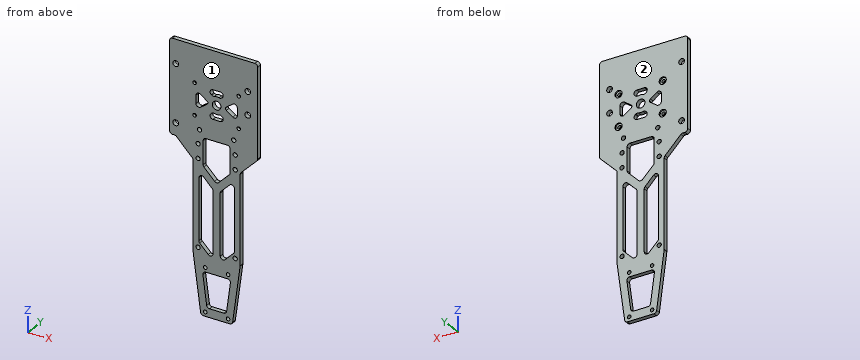
from build123d import *

# Parameters (mm, degrees)
SKETCH_1_R          = 1.25
SKETCH_1_R_2        = 1.5
EXTRUDE_1_DEPTH     = 3
CUT_EXTRUDE_1_DEPTH = 10
FILLET_1_R          = 2
SKETCH_3_R          = 2
CUT_EXTRUDE_2_DEPTH = 185.303255533
SKETCH_5_R          = 1.25
CUT_EXTRUDE_3_DEPTH = 185.303255533
SKETCH_6_R          = 3
CUT_EXTRUDE_4_DEPTH = 10
SKETCH_7_R          = 2.5
CUT_EXTRUDE_5_DEPTH = 1
FILLET_2_R          = 2
SKETCH_8_R          = 1.5
CUT_EXTRUDE_6_DEPTH = 10


with BuildPart() as part:
    # 草图1 → 凸台-拉伸1 (new body)
    with BuildSketch(Plane(origin=(0, 0, 0), x_dir=(1, 0, 0), z_dir=(0, 1, 0))):
        Polygon((11, 0), (-11, 0), (-16.5, -41.3), (-16.5, -104), (-28.8, -116.3), (-33, -116.3), (-33, -181.3), (28.8, -181.3), (28.8, -120.3), (28.8, -116.3), (16.5, -104), (16.5, -41.3), align=None)
        with Locations(Location((-8, -3, 0), (0, 0, 270))):
            Circle(SKETCH_1_R, mode=Mode.SUBTRACT)
        with Locations(Location((-8, -33, 0), (0, 0, 270))):
            Circle(SKETCH_1_R, mode=Mode.SUBTRACT)
        with Locations(Location((8, -33, 0), (0, 0, 90))):
            Circle(SKETCH_1_R, mode=Mode.SUBTRACT)
        with Locations(Location((8, -3, 0), (0, 0, 90))):
            Circle(SKETCH_1_R, mode=Mode.SUBTRACT)
        with Locations(Location((-13, -45.3, 0), (0, 0, 270))):
            Circle(SKETCH_1_R_2, mode=Mode.SUBTRACT)
        with Locations(Location((-13, -105.3, 0), (0, 0, 270))):
            Circle(SKETCH_1_R_2, mode=Mode.SUBTRACT)
        with Locations(Location((-13, -115.3, 0), (0, 0, 270))):
            Circle(SKETCH_1_R_2, mode=Mode.SUBTRACT)
        with Locations(Location((13, -115.3, 0), (0, 0, 90))):
            Circle(SKETCH_1_R_2, mode=Mode.SUBTRACT)
        with Locations(Location((13, -105.3, 0), (0, 0, 90))):
            Circle(SKETCH_1_R_2, mode=Mode.SUBTRACT)
        with Locations(Location((13, -45.3, 0), (0, 0, 90))):
            Circle(SKETCH_1_R_2, mode=Mode.SUBTRACT)
    extrude(amount=EXTRUDE_1_DEPTH)

    # 草图2 → 切除-拉伸1 (cut)
    with BuildSketch(Plane(origin=(0, 3, 0), x_dir=(1, 0, 0), z_dir=(0, 1, 0))):
        Polygon((6.754889433, -6), (-6.754889433, -6), (-9.951015341, -30), (9.951015341, -30), align=None)
        Polygon((12.5, -97.228932188), (2.5, -87.228932188), (2.5, -39.042640687), (12.5, -49.042640687), align=None)
        Polygon((-12.5, -49.042640687), (-2.5, -39.042640687), (-2.5, -87.228932188), (-12.5, -97.228932188), align=None)
        Polygon((-9.5, -101.3), (0, -91.8), (9.5, -101.3), (9.5, -120.3), (-9.5, -120.3), align=None)
    extrude(amount=-CUT_EXTRUDE_1_DEPTH, mode=Mode.SUBTRACT)

    # 圆角1
    fillet_1_edges = [part.edges().sort_by_distance(p)[0] for p in [
        (-9.951015341, 1.5, 30),
        (-6.754889433, 1.5, 6),
        (6.754889433, 1.5, 6),
        (9.951015341, 1.5, 30),
        (0, 1.5, 91.8),
        (9.5, 1.5, 101.3),
        (9.5, 1.5, 120.3),
        (-9.5, 1.5, 120.3),
        (-9.5, 1.5, 101.3),
        (12.5, 1.5, 49.042640687),
        (12.5, 1.5, 97.228932188),
        (2.5, 1.5, 87.228932188),
        (2.5, 1.5, 39.042640687),
        (-12.5, 1.5, 97.228932188),
        (-12.5, 1.5, 49.042640687),
        (-2.5, 1.5, 39.042640687),
        (-2.5, 1.5, 87.228932188),
        (-11, 1.5, 0),
        (11, 1.5, 0),
        (16.5, 1.5, 41.3),
        (16.5, 1.5, 104),
        (28.8, 1.5, 116.3),
        (28.8, 1.5, 181.3),
        (-33, 1.5, 181.3),
        (-33, 1.5, 116.3),
        (-28.8, 1.5, 116.3),
        (-16.5, 1.5, 104),
        (-16.5, 1.5, 41.3),
    ]]
    fillet(fillet_1_edges, radius=FILLET_1_R)

    # 草图3 → 切除-拉伸2 (cut, through all)
    with BuildSketch(Plane.XZ):
        with Locations(Location((-28.7, 164.8, 0), (0, 0, 270))):
            Circle(SKETCH_3_R)
        with Locations(Location((-28.7, 124.8, 0), (0, 0, 270))):
            Circle(SKETCH_3_R)
        with Locations(Location((21.8, 160.8, 0), (0, 0, 270))):
            Circle(SKETCH_3_R)
        with Locations(Location((21.8, 144.8, 0), (0, 0, 270))):
            Circle(SKETCH_3_R)
    extrude(amount=-CUT_EXTRUDE_2_DEPTH, mode=Mode.SUBTRACT)

    # 草图5 → 切除-拉伸3 (cut, through all)
    with BuildSketch(Plane(origin=(0, 3, 0), x_dir=(1, 0, 0), z_dir=(0, 1, 0))):
        with Locations(Location((15.5, -133.8, 0), (0, 0, 270))):
            Circle(SKETCH_5_R)
        with Locations(Location((-15.5, -133.8, 0), (0, 0, 270))):
            Circle(SKETCH_5_R)
        with Locations(Location((-15.5, -155.8, 0), (0, 0, 270))):
            Circle(SKETCH_5_R)
        with Locations(Location((15.5, -155.8, 0), (0, 0, 270))):
            Circle(SKETCH_5_R)
    extrude(amount=-CUT_EXTRUDE_3_DEPTH, mode=Mode.SUBTRACT)

    # 草图6 → 切除-拉伸4 (cut)
    with BuildSketch(Plane(origin=(0, 3, 0), x_dir=(1, 0, 0), z_dir=(0, 1, 0))):
        with BuildLine():
            Line((8.907296961, -134.8), (-8.907296961, -134.8))
            Line((-8.907296961, -134.8), (-2.501258408, -139.346220909))
            ThreePointArc((-2.501258408, -139.346220909), (0, -138.8), (2.501258408, -139.346220909))
            Line((2.501258408, -139.346220909), (8.907296961, -134.8))
        make_face()
        with BuildLine():
            Line((14.5, -151.411630102), (14.5, -138.188369898))
            Line((14.5, -138.188369898), (5.973740444, -144.239263777))
            ThreePointArc((5.973740444, -144.239263777), (5.993431516, -144.51932462), (6, -144.8))
            ThreePointArc((6, -144.8), (5.993431516, -145.08067538), (5.973740444, -145.360736223))
            Line((5.973740444, -145.360736223), (14.5, -151.411630102))
        make_face()
        with BuildLine():
            Line((-2.501258408, -150.253779091), (-8.907296961, -154.8))
            Line((-8.907296961, -154.8), (8.907296961, -154.8))
            Line((8.907296961, -154.8), (2.501258408, -150.253779091))
            ThreePointArc((2.501258408, -150.253779091), (0, -150.8), (-2.501258408, -150.253779091))
        make_face()
        with BuildLine():
            Line((-5.973740444, -144.239263777), (-14.5, -138.188369898))
            Line((-14.5, -138.188369898), (-14.5, -151.411630102))
            Line((-14.5, -151.411630102), (-5.973740444, -145.360736223))
            ThreePointArc((-5.973740444, -145.360736223), (-6, -144.8), (-5.973740444, -144.239263777))
        make_face()
        with Locations(Location((0, -144.8, 0), (0, 0, 270))):
            Circle(SKETCH_6_R)
    extrude(amount=-CUT_EXTRUDE_4_DEPTH, mode=Mode.SUBTRACT)

    # 草图7 → 切除-拉伸5 (cut)
    with BuildSketch(Plane(origin=(0, 3, 0), x_dir=(1, 0, 0), z_dir=(0, 1, 0))):
        with Locations(Location((15.5, -133.8, 0), (0, 0, 270))):
            Circle(SKETCH_7_R)
        with Locations(Location((-15.5, -133.8, 0), (0, 0, 270))):
            Circle(SKETCH_7_R)
        with Locations(Location((-15.5, -155.8, 0), (0, 0, 270))):
            Circle(SKETCH_7_R)
        with Locations(Location((15.5, -155.8, 0), (0, 0, 270))):
            Circle(SKETCH_7_R)
    extrude(amount=-CUT_EXTRUDE_5_DEPTH, mode=Mode.SUBTRACT)

    # 圆角2
    # the kernel refuses this fillet: 2 mm, written as the material it adds along each edge
    with BuildSketch(Plane(origin=(-2.501258408, 3, 150.253779091), x_dir=(-0.8155071447352907, 0, 0.5787470059410188), z_dir=(0, -1, 0)), Plane(origin=(5.973740444, 3, 145.360736223), x_dir=(0.8155071447351953, 0, 0.5787470059411531), z_dir=(0, -1, 0)), Plane(origin=(-5.973740444, 3, 144.239263777), x_dir=(-0.8155071447351933, 0, -0.578747005941156), z_dir=(0, -1, 0)), Plane(origin=(2.501258408, 3, 139.346220909), x_dir=(0.8155071447352105, 0, -0.5787470059411318), z_dir=(0, -1, 0))) as fillet_2_piece_1:
        with BuildLine():
            CenterArc((1.048845576, -2), FILLET_2_R, 90, 51.317812547)
            ThreePointArc((-0.512403924, -0.75), (-0.241988966, -0.384710393), (0, 0))
            Line((0, 0), (1.048845576, 0))
        make_face()
    extrude(amount=3)
    with BuildSketch(Plane(origin=(2.501258408, 3, 150.253779091), x_dir=(0.8155071447352289, 0, 0.578747005941106), z_dir=(0, -1, 0)), Plane(origin=(5.973740444, 3, 144.239263777), x_dir=(0.815507144735187, 0, -0.5787470059411648), z_dir=(0, -1, 0)), Plane(origin=(-5.973740444, 3, 145.360736223), x_dir=(-0.8155071447352036, 0, 0.5787470059411416), z_dir=(0, -1, 0)), Plane(origin=(-2.501258408, 3, 139.346220909), x_dir=(-0.8155071447352954, 0, -0.5787470059410122), z_dir=(0, -1, 0))) as fillet_2_piece_2:
        with BuildLine():
            CenterArc((1.048845576, 2), FILLET_2_R, 218.682187453, 51.317812547)
            ThreePointArc((-0.512403924, 0.75), (-0.241988966, 0.384710393), (0, 0))
            Line((0, 0), (1.048845576, 0))
        make_face()
    extrude(amount=3)
    with BuildSketch(Plane(origin=(8.907296961, 3, 154.8), x_dir=(-1, 0, 0), z_dir=(0, -1, 0)), Plane(origin=(-8.907296961, 3, 154.8), x_dir=(0.8155071447352168, 0, -0.578747005941123), z_dir=(0, -1, 0)), Plane(origin=(-8.907296961, 3, 134.8), x_dir=(1, 0, 0), z_dir=(0, -1, 0)), Plane(origin=(8.907296961, 3, 134.8), x_dir=(-0.815507144735218, 0, 0.5787470059411214), z_dir=(0, -1, 0))) as fillet_2_piece_3:
        with BuildLine():
            CenterArc((FILLET_2_R * 3.13696161898, FILLET_2_R), FILLET_2_R, 125.362461887, 144.637538113)
            Line((FILLET_2_R * 2.55821461304, FILLET_2_R * 1.81550714474), (0, 0))
            Line((0, 0), (FILLET_2_R * 3.13696161898, 0))
        make_face()
    extrude(amount=3)
    with BuildSketch(Plane(origin=(14.5, 3, 138.188369898), x_dir=(0, 0, 1), z_dir=(0, -1, 0)), Plane(origin=(14.5, 3, 151.411630102), x_dir=(-0.8155071447352171, 0, -0.5787470059411224), z_dir=(0, -1, 0)), Plane(origin=(-14.5, 3, 151.411630102), x_dir=(0, 0, -1), z_dir=(0, -1, 0)), Plane(origin=(-14.5, 3, 138.188369898), x_dir=(0.8155071447352167, 0, 0.578747005941123), z_dir=(0, -1, 0))) as fillet_2_piece_4:
        with BuildLine():
            CenterArc((FILLET_2_R * 1.93590824573, FILLET_2_R), FILLET_2_R, 144.637538113, 125.362461887)
            Line((FILLET_2_R * 1.12040110099, FILLET_2_R * 1.57874700594), (0, 0))
            Line((0, 0), (FILLET_2_R * 1.93590824573, 0))
        make_face()
    extrude(amount=3)

    # 草图8 → 切除-拉伸6 (cut)
    with BuildSketch(Plane(origin=(0, 3, 0), x_dir=(1, 0, 0), z_dir=(0, 1, 0))):
        with Locations(Location((12, -125.05, 0), (0, 0, 270))):
            Circle(SKETCH_8_R)
        with Locations(Location((-12, -125.05, 0), (0, 0, 270))):
            Circle(SKETCH_8_R)
    extrude(amount=-CUT_EXTRUDE_6_DEPTH, mode=Mode.SUBTRACT)


solid = part.part
Check sheet for the modelled part. Datum: model origin and axes. Units: mm. Face numbers are marked on the shaded views. Coordinates: 2 decimals unless noted, no trailing zeros. Loops run counter-clockwise (first coordinate to the right, second up) from the corner with the lowest first, then second, coordinate; pieces in that order, holes last. Notation, with made-up numbers: (-37.5, 82.25) -> (-20.5, 82.25) arc R32 cw to (-20.5, 110.25) -> close; hole circle Ø7 at (13, 14.25). An arc over 180 degrees is marked (long way). Answer in a Markdown table with one row per item.
1. Sectioned sample at D-D, the plane x = -22. Record the boundary of the cut face in (y, z), then the cut area to 3 significant figures.
Check values:
| item | result |
|---|---|
| outline | (0, 109.5) -> (3, 109.5) -> (3, 181.3) -> (0, 181.3) -> close |
| area | 215 mm2 |
2. Material ranges on line 1 along X through (y, z) = (2.85, 133.8); line 2 along X through (y, z) = (2.4, 86); line 3 along X through (y, z) = (1.8, 164.8), recorded low to high. Write a range as [from, to].
Check values:
| item | result |
|---|---|
| line 1 | x = [-33, -18], [-13, 13], [18, 28.8] |
| line 2 | x = [-16.5, -12.5], [-2.5, 2.5], [12.5, 16.5] |
| line 3 | x = [-33, -30.7], [-26.7, 28.8] |
3. Go/stop test with a flat-tipped pin: pin 1 (1.5 mm diameter, centred on y = 2.5, z = 19, fed in from -X). Record where the tip stops, or that it passes through.
Check values:
| item | result |
|---|---|
| pin 1 | stops at x = -13.63 |
4. Sectioned sample at A-A, the plane x = 21.8. Record the boundary of the cut face in (y, z), then the cut area to 3 significant figures.
Check values:
| item | result |
|---|---|
| outline | (0, 109.3) -> (3, 109.3) -> (3, 142.8) -> (0, 142.8) -> close; (0, 146.8) -> (3, 146.8) -> (3, 158.8) -> (0, 158.8) -> close; (0, 162.8) -> (3, 162.8) -> (3, 181.3) -> (0, 181.3) -> close |
| area | 192 mm2 |
5. Sectioned sample at C-C, the plane y = 1.3. Give the number of separate pieces and of enclosed holes in the cut face, then the cut area to 3 significant figures.
Check values:
| item | result |
|---|---|
| separate pieces | 1 |
| enclosed holes | 29 |
| area | 5,630 mm2 |
6. Sectioned sample at B-B, the plane z = 17. Record the boundary of the cut face in (x, y).
Check values:
| item | result |
|---|---|
| outline | (-13.26, 0) -> (-8.22, 0) -> (-8.22, 3) -> (-13.26, 3) -> close; (8.22, 0) -> (13.26, 0) -> (13.26, 3) -> (8.22, 3) -> close |
7. Release check for a two-part mould opening along Y. For the marked faces 1 and 2 record: released by +Y, released by -Y, zero draft, split by the parting line, or undercut.
Check values:
| item | result |
|---|---|
| face 1 | released by -Y |
| face 2 | released by +Y |
